Part model, mm, in its own coordinate system. A direction names the side the tool comes from. Coordinates: 2 decimals unless noted, no trailing zeros. Write each loop counter-clockwise with the first axis right and the second up, starting at its lowest first coordinate (ties: lowest second). Pieces come first, ordered by that corner, then holes. Notation, with made-up numbers: (-14, 20) - (41, 20) arc R26 cw to (41, 52) - close; hole circle Ø11 at (-27.5, 36). An arc over 180 degrees is marked (long way). Use a Markdown table: item, result.
```python
from build123d import *

# Parameters (mm, degrees)
F0_W     = 32
F0_H     = 11.5
F1_DEPTH = 3
F2_R     = 2
F3_W     = 13
F3_H     = 3.5
F4_DEPTH = 3.001
F5_R     = 2


with BuildPart() as f1:
    # F0 (on Top) → F1 (new body)
    with BuildSketch(Plane.XY):
        with Locations((0, 5.75)):
            Rectangle(F0_W, F0_H)
    extrude(amount=F1_DEPTH)

    # F2
    f2_edges = [f1.edges().sort_by_distance(p)[0] for p in [
        (-16, 11.5, 1.5),
        (16, 11.5, 1.5),
    ]]
    fillet(f2_edges, radius=F2_R)

    # F3 (on face) → F4 (cut, through all)
    with BuildSketch(Plane.XY.offset(3)):
        with Locations((0, 1.75)):
            Rectangle(F3_W, F3_H)
    extrude(amount=-F4_DEPTH, mode=Mode.SUBTRACT)

    # F5
    f5_edges = [f1.edges().sort_by_distance(p)[0] for p in [
        (-6.5, 3.5, 1.5),
        (6.5, 3.5, 1.5),
    ]]
    fillet(f5_edges, radius=F5_R)


solid = f1.part
```
Item 1: Band-saw the part on A-A, the plane z = 0.6. Give the cut face in (x, y), then the cut area to 4 significant figures.
From the geometry:
| item | result |
|---|---|
| outline | (-16, 0) - (-6.5, 0) - (-6.5, 1.5) arc R2 cw to (-4.5, 3.5) - (4.5, 3.5) arc R2 cw to (6.5, 1.5) - (6.5, 0) - (16, 0) - (16, 9.5) arc R2 ccw to (14, 11.5) - (-14, 11.5) arc R2 ccw to (-16, 9.5) - close |
| area | 322.5 mm^2 |
Item 2: Two-plate mould, pull along X, no slides. Class faces 3 (the face through (-6.5, 1, 2)), 4 (the face through (6.5, 1, 2)), 5 (the face through (-11, 0, 1)), 6 (the face through (-16, 5, 1)): pulls with the +X half, pulls with the -X half, needs draft (parallel to the pull), parting line crosses it, or undercut.
From the geometry:
| item | result |
|---|---|
| face 3 | undercut |
| face 4 | undercut |
| face 5 | needs draft |
| face 6 | pulls with the -X half |
Item 3: Band-saw the part on B-B, the plane x = 0.5. Give the cut face in (y, z).
From the geometry:
| item | result |
|---|---|
| outline | (3.5, 0) - (11.5, 0) - (11.5, 3) - (3.5, 3) - close |
Item 4: Band-saw the part on C-C, the plane y = 10.75. Give the cut face in (x, z).
From the geometry:
| item | result |
|---|---|
| outline | (-15.56, 0) - (15.56, 0) - (15.56, 3) - (-15.56, 3) - close |
Item 5: Drop a flat-ended pin along its axis: P1, Ø1, axis at x = 0, z = 1, coming from the -Y side. Give the stop position or say it passes through.
From the geometry:
| item | result |
|---|---|
| P1 | y = 3.5 |
Item 6: Which spindle directions (+Z, -Z, +X, -X, +Y, -Y) get a long thin tool onto all of the face, cutting with end or side? Do faces 1 (the face through (-15.43, 10.9, 1.52)), 2 (the face through (5.93, 2.9, 1.48)). Say none if no direction does.
From the geometry:
| item | result |
|---|---|
| face 1 | +Z, -Z, -X, +Y |
| face 2 | +Z, -Z, -Y |
Item 7: Drill centre lines: probe 1 along X at (y, z) = (0.5, 2.6); probe 2 along Y at (x, z) = (-1.5, 2.8); probe 3 along Y at (x, z) = (-6, 2.6). Where is each one in solid material? Low to high.
From the geometry:
| item | result |
|---|---|
| probe 1 | -16 to -6.5, 6.5 to 16 |
| probe 2 | 3.5 to 11.5 |
| probe 3 | 2.82 to 11.5 |
